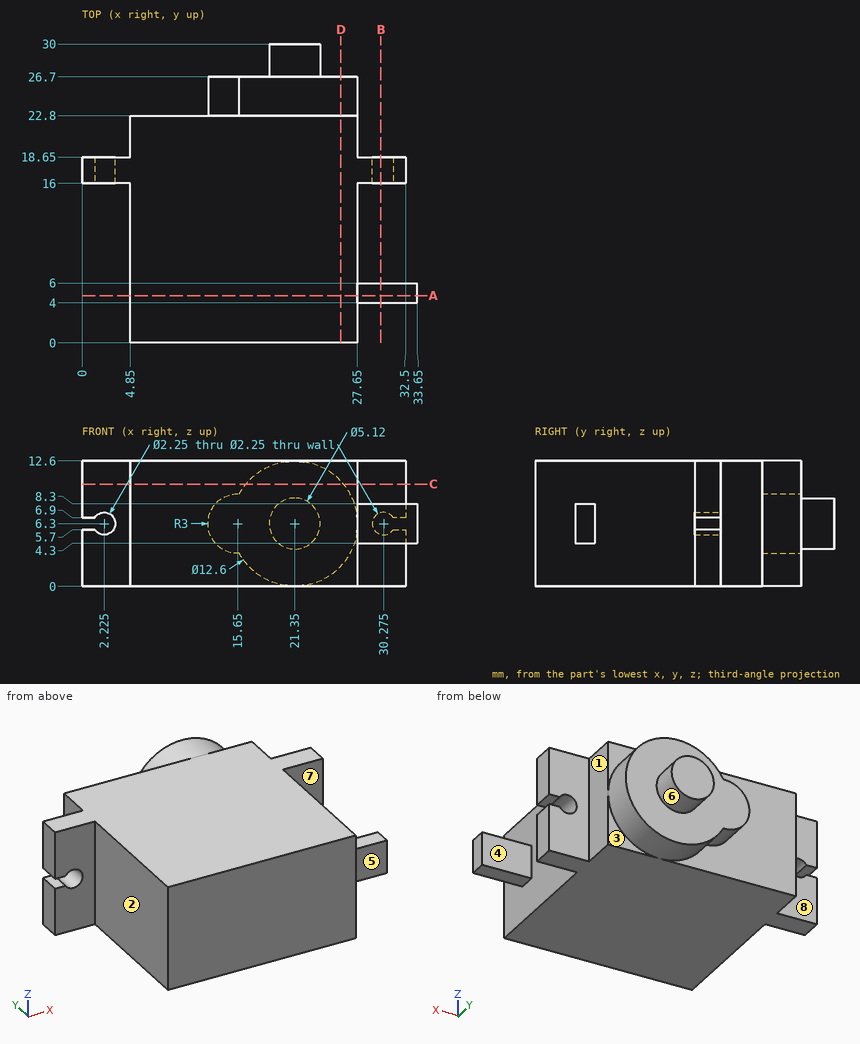
The figure shows three views and two pictorial views of one solid part (mm, origin at its lowest corner). Answer the questions. A direction names the side the tool comes from. Give positions to 0.01 mm unless a question says otherwise; leave off trailing zeros. Write each loop counter-clockwise with the first axis right and the second up, starting at its lowest first coordinate (ties: lowest second). Pieces come first, ordered by that corner, then holes. Notation, with made-up numbers: (-5, -22.75) - (3, -22.75) arc R30 ccw to (3, 16.25) - close; hole circle Ø10 at (16.5, 2). An arc over 180 degrees is marked (long way). Use one line per item in the form item = value.
1. A cutting plane is placed at D-D (x = 26). Write down the section's boundary in (y, z), and give its area (3 significant figures).
Filled in:
outline = (0, 0) - (22.8, 0) - (22.8, 2.05) - (26.7, 2.05) - (26.7, 10.55) - (22.8, 10.55) - (22.8, 12.6) - (0, 12.6) - close
area = 320 mm^2
2. Consider L1, parallel to Y at x = 32, z = 9; L2, parallel to Y at x = 22, z = 3; L3, parallel to X at y = 4, z = 9.25. Determine where each line is inside the solid, lowest interval first.
Filled in:
L1 = 16 to 18.65
L2 = 0 to 26.7
L3 = 4.85 to 27.65
3. A cutting plane is placed at A-A (y = 4.75). Write down the section's boundary in (x, z), and give its area (3 significant figures).
Filled in:
outline = (4.85, 0) - (27.65, 0) - (27.65, 4.3) - (33.65, 4.3) - (33.65, 8.3) - (27.65, 8.3) - (27.65, 12.6) - (4.85, 12.6) - close
area = 311 mm^2
4. A cutting plane is placed at C-C (z = 10.25). Write down the section's boundary in (x, y), and give its area (3 significant figures).
Filled in:
outline = (0, 16) - (4.85, 16) - (4.85, 0) - (27.65, 0) - (27.65, 16) - (32.5, 16) - (32.5, 18.65) - (27.65, 18.65) - (27.65, 22.8) - (26.26, 22.8) - (26.26, 26.7) - (16.44, 26.7) - (16.44, 22.8) - (4.85, 22.8) - (4.85, 18.65) - (0, 18.65) - close
area = 584 mm^2
5. Each of these flat-tipped pins is pushed along its axis until it touches: pin 1 Ø3 at (y, z) = (11, 1.5) entering from +X; pin 2 Ø1.6 at (x, y) = (30.5, 5) entering from -Z; pin 3 Ø3 at (y, z) = (4, 5) entering from -X. Where does it stop, or does it pass through?
Filled in:
pin_1 = 27.65
pin_2 = 4.3
pin_3 = 4.85
6. Determine the mould class of the marked faces 6, 7 and 8 for opening direction Y: released by +Y, released by -Y, zero draft, split by the parting line, or undercut.
Filled in:
face_6 = zero draft
face_7 = undercut
face_8 = released by +Y
7. A cutting plane is placed at B-B (x = 30). Write down the section's boundary in (y, z), and give its area (3 significant figures).
Filled in:
outline = (4, 4.3) - (6, 4.3) - (6, 8.3) - (4, 8.3) - close; (16, 0) - (18.65, 0) - (18.65, 5.21) - (16, 5.21) - close; (16, 7.39) - (18.65, 7.39) - (18.65, 12.6) - (16, 12.6) - close
area = 35.6 mm^2
8. For the marked faces 1, 2, 3, 4 and 5, determine the directions among +Z, -Z, +X, -X, +Y, -Y from which every point of the face is accessible in a straight line to the end or side of a thin tool.
Filled in:
face_1 = +Z, -Z, +X, +Y
face_2 = +Z, -Z, -X, -Y
face_3 = -Z, +X, +Y
face_4 = +Z, -Z, +X
face_5 = +Z, -Z, +X, -Y
